```python
from build123d import *

# Parameters (mm, degrees)
F0_W      = 31.8
F0_H      = 31.8
F0_R      = 6.5
F1_DEPTH  = 3
F2_DEPTH  = 10
F0_W_2    = 45.8
F0_H_2    = 45.8
F3_DEPTH  = 13
F5_START  = -5
F5_DEPTH  = 3
F6_D      = 6
F6_DEPTH  = 1.5
F6_TIP    = 1.8025818571
F7_D      = 3.3
F7_DEPTH  = 10
F7_START  = 2.3111618
F7_TIP    = 0.9914200214
F9_START  = -5
F9_DEPTH  = 3
F11_START = -5
F11_DEPTH = 3
F12_D     = 3.3
F12_DEPTH = 10
F12_TIP   = 0.9914200214
F13_D     = 6
F13_DEPTH = 1.5
F13_TIP   = 1.8025818571
F14_D     = 6
F14_DEPTH = 1.5
F14_TIP   = 1.8025818571
F15_D     = 3.3
F15_DEPTH = 10
F15_START = 2.3111618
F15_TIP   = 0.9914200214
F17_START = -5
F17_DEPTH = 3
F18_D     = 3.3
F18_DEPTH = 10
F18_TIP   = 0.9914200214
F19_D     = 6
F19_DEPTH = 1.5
F19_TIP   = 1.8025818571
F20_R     = 2
F21_D     = 6.5278
F21_DEPTH = 15.81
F21_TIP   = 1.9611489744


with BuildPart() as f1:
    # F0 (on Front) → F1 (new body)
    with BuildSketch(Plane.XZ):
        Rectangle(F0_W, F0_H)
        Circle(F0_R, mode=Mode.SUBTRACT)
    extrude(amount=F1_DEPTH)

    # F0 (on Front) → F2 (join)
    with BuildSketch(Plane.XZ):
        Circle(F0_R)
    extrude(amount=F2_DEPTH)

    # F0 (on Front) → F3 (join)
    with BuildSketch(Plane.XZ):
        Rectangle(F0_W_2, F0_H_2)
        Rectangle(F0_W, F0_H, mode=Mode.SUBTRACT)
    extrude(amount=F3_DEPTH)

    # F4 (on face) → F5 (cut)
    with BuildSketch(Plane(origin=(0, 0, -22.9), x_dir=(1, 0, 0), z_dir=(0, 0, -1)).offset(F5_START)):
        Polygon((-6.8256842194, 5.1), (-5.1513684387, 8), (-6.8256842194, 10.9), (-10.1743157806, 10.9), (-11.8486315613, 8), (-10.1743157806, 5.1), align=None)
        Polygon((10.1743157806, 5.1), (11.8486315613, 8), (10.1743157806, 10.9), (6.8256842194, 10.9), (5.1513684387, 8), (6.8256842194, 5.1), align=None)
    extrude(amount=-F5_DEPTH, mode=Mode.SUBTRACT)

    # F6
    with Locations(Plane(origin=(0, 0, -22.9), x_dir=(1, 0, 0), z_dir=(0, 0, -1))):
        with Locations((-8.5, 8), (8.5, 8)):
            Hole(F6_D / 2, depth=F6_DEPTH)
            with Locations((0, 0, -(F6_DEPTH + F6_TIP / 2))):  # 118° drill point
                Cone(0, F6_D / 2, F6_TIP, mode=Mode.SUBTRACT)

    # F7
    # its depths count from where the whole tool has entered the part; down to there all is cleared
    with Locations(Plane(origin=(0, 0, -22.9), x_dir=(1, 0, 0), z_dir=(0, 0, -1)).offset(-F7_START)):
        with Locations((-8.5, 8), (8.5, 8)):
            Hole(F7_D / 2, depth=F7_DEPTH)
            with Locations((0, 0, -(F7_DEPTH + F7_TIP / 2))):  # 118° drill point
                Cone(0, F7_D / 2, F7_TIP, mode=Mode.SUBTRACT)

    # F8 (on face) → F9 (cut)
    with BuildSketch(Plane.YZ.offset(22.9).offset(F9_START)):
        Polygon((-5.1, -6.8256842194), (-8, -5.1513684387), (-10.9, -6.8256842194), (-10.9, -10.1743157806), (-8, -11.8486315613), (-5.1, -10.1743157806), align=None)
        Polygon((-5.1, 10.1743157806), (-8, 11.8486315613), (-10.9, 10.1743157806), (-10.9, 6.8256842194), (-8, 5.1513684387), (-5.1, 6.8256842194), align=None)
    extrude(amount=-F9_DEPTH, mode=Mode.SUBTRACT)

    # F10 (on face) → F11 (cut)
    with BuildSketch(Plane.XY.offset(22.9).offset(F11_START)):
        Polygon((6.8256842194, -5.1), (5.1513684387, -8), (6.8256842194, -10.9), (10.1743157806, -10.9), (11.8486315613, -8), (10.1743157806, -5.1), align=None)
        Polygon((-6.8256842194, -5.1), (-10.1743157806, -5.1), (-11.8486315613, -8), (-10.1743157806, -10.9), (-6.8256842194, -10.9), (-5.1513684387, -8), align=None)
    extrude(amount=-F11_DEPTH, mode=Mode.SUBTRACT)

    # F12
    with Locations(Plane.XY.offset(22.9)):
        with Locations((8.5, -8), (-8.5, -8)):
            Hole(F12_D / 2, depth=F12_DEPTH)
            with Locations((0, 0, -(F12_DEPTH + F12_TIP / 2))):  # 118° drill point
                Cone(0, F12_D / 2, F12_TIP, mode=Mode.SUBTRACT)

    # F13
    with Locations(Plane.XY.offset(22.9)):
        with Locations((8.5, -8), (-8.5, -8)):
            Hole(F13_D / 2, depth=F13_DEPTH)
            with Locations((0, 0, -(F13_DEPTH + F13_TIP / 2))):  # 118° drill point
                Cone(0, F13_D / 2, F13_TIP, mode=Mode.SUBTRACT)

    # F14
    with Locations(Plane.YZ.offset(22.9)):
        with Locations((-8, -8.5), (-8, 8.5)):
            Hole(F14_D / 2, depth=F14_DEPTH)
            with Locations((0, 0, -(F14_DEPTH + F14_TIP / 2))):  # 118° drill point
                Cone(0, F14_D / 2, F14_TIP, mode=Mode.SUBTRACT)

    # F15
    # its depths count from where the whole tool has entered the part; down to there all is cleared
    with Locations(Plane.YZ.offset(22.9).offset(-F15_START)):
        with Locations((-8, -8.5), (-8, 8.5)):
            Hole(F15_D / 2, depth=F15_DEPTH)
            with Locations((0, 0, -(F15_DEPTH + F15_TIP / 2))):  # 118° drill point
                Cone(0, F15_D / 2, F15_TIP, mode=Mode.SUBTRACT)

    # F16 (on face) → F17 (cut)
    with BuildSketch(Plane(origin=(-22.9, 0, 0), x_dir=(0, -1, 0), z_dir=(-1, 0, 0)).offset(F17_START)):
        Polygon((5.1, 10.1743157806), (5.1, 6.8256842194), (8, 5.1513684387), (10.9, 6.8256842194), (10.9, 10.1743157806), (8, 11.8486315613), align=None)
        Polygon((5.1, -6.8256842194), (5.1, -10.1743157806), (8, -11.8486315613), (10.9, -10.1743157806), (10.9, -6.8256842194), (8, -5.1513684387), align=None)
    extrude(amount=-F17_DEPTH, mode=Mode.SUBTRACT)

    # F18
    with Locations(Plane(origin=(-22.9, 0, 0), x_dir=(0, -1, 0), z_dir=(-1, 0, 0))):
        with Locations((8, 8.5), (8, -8.5)):
            Hole(F18_D / 2, depth=F18_DEPTH)
            with Locations((0, 0, -(F18_DEPTH + F18_TIP / 2))):  # 118° drill point
                Cone(0, F18_D / 2, F18_TIP, mode=Mode.SUBTRACT)

    # F19
    with Locations(Plane(origin=(-22.9, 0, 0), x_dir=(0, -1, 0), z_dir=(-1, 0, 0))):
        with Locations((8, 8.5), (8, -8.5)):
            Hole(F19_D / 2, depth=F19_DEPTH)
            with Locations((0, 0, -(F19_DEPTH + F19_TIP / 2))):  # 118° drill point
                Cone(0, F19_D / 2, F19_TIP, mode=Mode.SUBTRACT)

    # F20
    f20_edges = [f1.edges().sort_by_distance(p)[0] for p in [
        (22.9, -6.5, 22.9),
        (22.9, -6.5, -22.9),
        (-22.9, -6.5, -22.9),
        (-22.9, -6.5, 22.9),
    ]]
    fillet(f20_edges, radius=F20_R)

    # F21
    with Locations(Plane(origin=(0, 0, 0), x_dir=(1, 0, 0), z_dir=(0, 1, 0))):
        with Locations((0, 0)):
            Hole(F21_D / 2, depth=F21_DEPTH)
            with Locations((0, 0, -(F21_DEPTH + F21_TIP / 2))):  # 118° drill point
                Cone(0, F21_D / 2, F21_TIP, mode=Mode.SUBTRACT)


solid = f1.part
```
CAD build for the part. Positions are in the model's coordinates, mm. A direction names the side the tool comes from. Give positions to 0.01 mm unless a question says otherwise; leave off trailing zeros. Write each loop counter-clockwise with the first axis right and the second up, starting at its lowest first coordinate (ties: lowest second). Pieces come first, ordered by that corner, then holes. Notation, with made-up numbers: M 51,46.5 L 110,46.5 A24 cw 110,65.5 Z; hole C 28.25,29.5 d6. An arc over 180 degrees is marked long. Return JSON: item names as keys, results as strings. Group by question number.
(1) Band-saw the part on A-A (y = -4). Give the cut face in (x, z).
(2) Mould opens along Z. For faces 1 (the face through (0, -6, 22.9)), 2 (the face through (9.716, -9.115, -19.226)), 3 (the face through (-16.91, -6.53, 6)), 4 (the face through (-5.977, -9.43, -16.914)) say: pulls with the +Z half, pulls with the -Z half, needs draft (parallel to the pull), parting line crosses it, or undercut.
(3) Band-saw the part on C-C (x = 0). Give the cut face in (y, z).
(4) Drill centre lines: L1, parallel to Z at x = -19, y = -8; L2, parallel to X at y = -10.25, z = -6. Where is each one in solid material? Low to high. Write a range as [from, to].
(5) Band-saw the part on D-D (z = 17). Give the cut face in (x, y), and give its area (3 significant figures).
(6) Band-saw the part on B-B (z = -8.5). State how many separate pieces and enclosed holes the cut face has, and give its area (3 significant figures).
(7) 3-axis set-ups, long thin cutter, end or side, ignore diameter. For faces 5 (the face through (0, -6, -22.9)), 6 (the face through (-11.36, -7.1, 22.14)), 7 (the face through (-5.977, -6.57, 16.914)): which of +Z, -Z, +X, -X, +Y, -Y reach the whole face in a straight line?
(8) Flat gauge pins, fed straight in: pin 1 Ø3 at (x, y) = (8.5, -8) entering from +Z; pin 2 Ø5.5 at (y, z) = (-8, 8.5) entering from -X; pin 3 Ø5.5 at (x, y) = (-8.5, -8) entering from -Z. Where does each tip first touch, or does it go through?
Entries:
{
 "1": {"outline": "M -22.9,-20.9 A2 ccw -20.9,-22.9 L 20.9,-22.9 A2 ccw 22.9,-20.9 L 22.9,20.9 A2 ccw 20.9,22.9 L -20.9,22.9 A2 ccw -22.9,20.9 Z; C 0,0 d13; hole M -15.9,-15.9 L 15.9,-15.9 L 15.9,15.9 L -15.9,15.9 Z; hole C 0,0 d6.53"},
 "2": {"face 1": "pulls with the +Z half", "face 2": "needs draft", "face 3": "undercut", "face 4": "undercut"},
 "3": {"outline": "M -13,-22.9 L 0,-22.9 L 0,-3.26 L -10,-3.26 L -10,-6.5 L -3,-6.5 L -3,-15.9 L -13,-15.9 Z; M -13,15.9 L -3,15.9 L -3,6.5 L -10,6.5 L -10,3.26 L 0,3.26 L 0,22.9 L -13,22.9 Z"},
 "4": {"L1": "z = [-22.9, -10.15], [-6.85, 6.85], [10.15, 22.9]", "L2": "x = [-22.9, -15.9], [15.9, 22.9]"},
 "5": {"outline": "M -22.9,-13 L 22.9,-13 L 22.9,0 L -22.9,0 Z; hole M -11.85,-8 L -10.17,-10.9 L -6.83,-10.9 L -5.15,-8 L -6.83,-5.1 L -10.17,-5.1 Z; hole M 5.15,-8 L 6.83,-10.9 L 10.17,-10.9 L 11.85,-8 L 10.17,-5.1 L 6.83,-5.1 Z", "area": "537 mm^2"},
 "6": {"separate pieces": "3", "enclosed holes": "0", "area": "211 mm^2"},
 "7": {"face 5": "-Z, +X, -X, +Y, -Y", "face 6": "+Z", "face 7": "none"},
 "8": {"pin 1": "passes through", "pin 2": "stops at x = -21.25", "pin 3": "stops at z = -21.25"}
}
